The listing builds one solid part. Answer for the finished solid, in the listing's coordinates (mm). A direction names the side the tool comes from. Coordinates: 2 decimals unless noted, no trailing zeros. Write each loop counter-clockwise with the first axis right and the second up, starting at its lowest first coordinate (ties: lowest second). Pieces come first, ordered by that corner, then holes.
from build123d import *

# Parameters (mm, degrees)
SKETCH1_W           = 25
SKETCH1_H           = 24
BOSS_EXTRUDE1_DEPTH = 1.5
SKETCH2_W           = 8
SKETCH2_H           = 8
BOSS_EXTRUDE2_DEPTH = 2
SKETCH3_R           = 3.175
BOSS_EXTRUDE3_DEPTH = 3
SKETCH5_W           = 5
SKETCH5_H           = 20
BOSS_EXTRUDE4_DEPTH = 3
CUT_EXTRUDE1_REACH  = 20.035
SKETCH6_R           = 0.95


with BuildPart() as part:
    # Sketch1 → Boss-Extrude1 (new body)
    with BuildSketch(Plane(origin=(0, 0, 0), x_dir=(1, 0, 0), z_dir=(0, 1, 0))):
        Rectangle(SKETCH1_W, SKETCH1_H)
    extrude(amount=BOSS_EXTRUDE1_DEPTH)

    # Sketch2 → Boss-Extrude2 (add)
    with BuildSketch(Plane(origin=(0, 1.5, 0), x_dir=(1, 0, 0), z_dir=(0, 1, 0))):
        with Locations((1.5, 0)):
            Rectangle(SKETCH2_W, SKETCH2_H)
    extrude(amount=BOSS_EXTRUDE2_DEPTH)

    # Sketch3 → Boss-Extrude3 (add)
    with BuildSketch(Plane(origin=(0, 3.5, 0), x_dir=(1, 0, 0), z_dir=(0, 1, 0))):
        with Locations(Location((1.5, 0, 0), (0, 0, 270))):
            Circle(SKETCH3_R)
    extrude(amount=BOSS_EXTRUDE3_DEPTH)

    # Sketch5 → Boss-Extrude4 (add)
    with BuildSketch(Plane.XZ):
        with Locations((9.5, 0)):
            Rectangle(SKETCH5_W, SKETCH5_H)
    extrude(amount=BOSS_EXTRUDE4_DEPTH)

    # Sketch6 → Cut-Extrude1 (cut, up to next)
    with BuildSketch(Plane(origin=(0, 1.5, 0), x_dir=(1, 0, 0), z_dir=(0, 1, 0)), mode=Mode.PRIVATE) as cut_extrude1_sk1:
        with Locations(Location((-10.5, 10, 0), (0, 0, 270))):
            Circle(SKETCH6_R)
    cut_extrude1_tool1 = extrude(cut_extrude1_sk1.sketch, amount=-CUT_EXTRUDE1_REACH, mode=Mode.PRIVATE) & part.part
    # Sketch6 → Cut-Extrude1 (cut, up to next)
    with BuildSketch(Plane(origin=(0, 1.5, 0), x_dir=(1, 0, 0), z_dir=(0, 1, 0)), mode=Mode.PRIVATE) as cut_extrude1_sk2:
        with Locations(Location((1.5, 10, 0), (0, 0, 270))):
            Circle(SKETCH6_R)
    cut_extrude1_tool2 = extrude(cut_extrude1_sk2.sketch, amount=-CUT_EXTRUDE1_REACH, mode=Mode.PRIVATE) & part.part
    # Sketch6 → Cut-Extrude1 (cut, up to next)
    with BuildSketch(Plane(origin=(0, 1.5, 0), x_dir=(1, 0, 0), z_dir=(0, 1, 0)), mode=Mode.PRIVATE) as cut_extrude1_sk3:
        with Locations(Location((-10.5, -10, 0), (0, 0, 270))):
            Circle(SKETCH6_R)
    cut_extrude1_tool3 = extrude(cut_extrude1_sk3.sketch, amount=-CUT_EXTRUDE1_REACH, mode=Mode.PRIVATE) & part.part
    # Sketch6 → Cut-Extrude1 (cut, up to next)
    with BuildSketch(Plane(origin=(0, 1.5, 0), x_dir=(1, 0, 0), z_dir=(0, 1, 0)), mode=Mode.PRIVATE) as cut_extrude1_sk4:
        with Locations(Location((1.5, -10, 0), (0, 0, 270))):
            Circle(SKETCH6_R)
    cut_extrude1_tool4 = extrude(cut_extrude1_sk4.sketch, amount=-CUT_EXTRUDE1_REACH, mode=Mode.PRIVATE) & part.part
    add(cut_extrude1_tool1.solids().sort_by_distance((-10.5, 1.5, -10))[0], mode=Mode.SUBTRACT)
    add(cut_extrude1_tool2.solids().sort_by_distance((1.5, 1.5, -10))[0], mode=Mode.SUBTRACT)
    add(cut_extrude1_tool3.solids().sort_by_distance((-10.5, 1.5, 10))[0], mode=Mode.SUBTRACT)
    add(cut_extrude1_tool4.solids().sort_by_distance((1.5, 1.5, 10))[0], mode=Mode.SUBTRACT)


solid = part.part
1. Section A-A on x = 1.5 is taken. Give the vertices of the cut face in (y, z) (3 decimals).
Results found:
outline: (0, -12) - (1.5, -12) - (1.5, -10.95) - (0, -10.95) - close; (0, -9.05) - (1.5, -9.05) - (1.5, -4) - (3.5, -4) - (3.5, -3.175) - (6.5, -3.175) - (6.5, 3.175) - (3.5, 3.175) - (3.5, 4) - (1.5, 4) - (1.5, 9.05) - (0, 9.05) - close; (0, 10.95) - (1.5, 10.95) - (1.5, 12) - (0, 12) - close
2. Section B-B on z = -10.5 is taken. Give the vertices of the cut face in (x, y), then the cut area to 3 significant figures.
Results found:
outline: (-12.5, 0) - (-11.31, 0) - (-11.31, 1.5) - (-12.5, 1.5) - close; (-9.69, 0) - (0.69, 0) - (0.69, 1.5) - (-9.69, 1.5) - close; (2.31, 0) - (12.5, 0) - (12.5, 1.5) - (2.31, 1.5) - close
area: 32.7 mm2
3. A tool of negligible diameter and unlimited length cuts with its end or side. For faces 1 (the flat face through (1, 2, 4)), 2 (the flat face through (12, -1, 0)), 3 (the flat face through (1, 2, -4)), 4 (the flat face through (5.5, 2, 0)), 5 (the flat face through (9, -1, 10)), from which of +Z, -Z, +X, -X, +Y, -Y can it reach the whole face along a straight path? Write none if from no direction.
Results found:
face 1: +Z, +X, -X, +Y
face 2: +Z, -Z, +X, -Y
face 3: -Z, +X, -X, +Y
face 4: +Z, -Z, +X, +Y
face 5: +Z, +X, -X, -Y
4. Section D-D on x = -10.5 is taken. Give the vertices of the cut face in (y, z).
Results found:
outline: (0, -12) - (1.5, -12) - (1.5, -10.95) - (0, -10.95) - close; (0, -9.05) - (1.5, -9.05) - (1.5, 9.05) - (0, 9.05) - close; (0, 10.95) - (1.5, 10.95) - (1.5, 12) - (0, 12) - close
5. Section C-C on z = 0 is taken. Give the vertices of the cut face in (x, y) (3 decimals).
Results found:
outline: (-12.5, 0) - (7, 0) - (7, -3) - (12, -3) - (12, 0) - (12.5, 0) - (12.5, 1.5) - (5.5, 1.5) - (5.5, 3.5) - (4.675, 3.5) - (4.675, 6.5) - (-1.675, 6.5) - (-1.675, 3.5) - (-2.5, 3.5) - (-2.5, 1.5) - (-12.5, 1.5) - close
6. For a pull along X with two mould halves and no side action, classify faces 6 (the cylindrical face through (2.14, 0.76, -10.7)), 7 (the cylindrical face through (-1.6, 4.98, -0.69)), 8 (the cylindrical face through (-9.86, 0.76, -10.7)), 9 (the flat face through (7, -1, 0)) as pulls with the +X half, pulls with the -X half, needs draft (parallel to the pull), parting line crosses it, or undercut.
Results found:
face 6: undercut
face 7: parting line crosses it
face 8: undercut
face 9: pulls with the -X half
7. Find the intervals of material crossed by L1, parallel to X at y = 0.6, z = -10; L2, parallel to Y at x = -1.75, z = -7.5; L3, parallel to Z at x = -1.5, y = 3.25, in increasing order.
Results found:
L1: x = -12.5 to -11.45, -9.55 to 0.55, 2.45 to 12.5
L2: y = 0 to 1.5
L3: z = -4 to 4
8. Flat-ended cylindrical pins translate along their axes: P1, Ø12, axis at x = 5, z = -5, coming from the -Y side; P2, Ø1.7, axis at x = 1.5, z = 10, coming from the -Y side; P3, Ø3, axis at x = 1.5, z = -10, coming from the -Y side; P4, Ø0.9, axis at x = 9.5, y = -2, coming from the +Z side. Find the tip coordinate at first contact, or state that the pin passes through.
Results found:
P1: stops at y = -3
P2: passes through
P3: stops at y = 0
P4: stops at z = 10
